The listing builds one solid part. Answer for the finished solid, in the listing's coordinates (mm). Coordinates: 2 decimals unless noted, no trailing zeros. Loops run counter-clockwise (first coordinate to the right, second up) from the corner with the lowest first, then second, coordinate; pieces in that order, holes last. Notation, with made-up numbers: (-13.5, 55) - (19.5, 55) arc R19 ccw to (19.5, 90) - close; hole circle Ø8 at (5, -11). An arc over 180 degrees is marked (long way). Put each result on its own line as item: value.
```python
from build123d import *

# Parameters (mm, degrees)
F1_DEPTH = 6


with BuildPart() as f1:
    # F0 (on Right) → F1 (new body)
    with BuildSketch(Plane.YZ):
        Polygon((9.433792, 157.218419), (-47.5, 157.218419), (-47.5, 130.369142), (-32.5, 130.369142), (-32.5, 142.218419), (9.433792, 142.218419), align=None)
        Polygon((62.5, 157.218419), (9.433792, 157.218419), (9.433792, 142.218419), (47.5, 142.218419), (47.5, 129.836887), (62.5, 129.836887), align=None)
        Polygon((-32.5, 130.369142), (-47.5, 130.369142), (-47.5, -62.781581), (62.5, -62.781581), (62.5, 129.836887), (47.5, 129.836887), (47.5, 119.718419), (-32.5, 119.718419), align=None)
        Polygon((-22.5, -19.281581), (-22.5, -22.781581), (-22.5, -26.281581), (-32.5, -26.281581), (-32.5, -19.281581), align=None, mode=Mode.SUBTRACT)
        Polygon((12.5, -19.281581), (12.5, -22.781581), (12.5, -26.281581), (2.5, -26.281581), (2.5, -22.781581), (2.5, -19.281581), align=None, mode=Mode.SUBTRACT)
        Polygon((37.5, -22.781581), (37.5, -19.281581), (47.5, -19.281581), (47.5, -26.281581), (37.5, -26.281581), align=None, mode=Mode.SUBTRACT)
        Polygon((-22.5, 55.718419), (-22.5, 52.218419), (-22.5, 48.718419), (-32.5, 48.718419), (-32.5, 55.718419), align=None, mode=Mode.SUBTRACT)
        Polygon((-22.5, 102.218419), (-22.5, 98.718419), (-32.5, 98.718419), (-32.5, 105.718419), (-22.5, 105.718419), align=None, mode=Mode.SUBTRACT)
        Polygon((12.5, 55.718419), (12.5, 52.218419), (12.5, 48.718419), (2.5, 48.718419), (2.5, 52.218419), (2.5, 55.718419), align=None, mode=Mode.SUBTRACT)
        Polygon((37.5, 52.218419), (37.5, 55.718419), (47.5, 55.718419), (47.5, 48.718419), (37.5, 48.718419), align=None, mode=Mode.SUBTRACT)
        Polygon((2.5, 98.718419), (2.5, 102.218419), (2.5, 105.718419), (12.5, 105.718419), (12.5, 102.218419), (12.5, 98.718419), align=None, mode=Mode.SUBTRACT)
        Polygon((37.5, 98.718419), (37.5, 102.218419), (37.5, 105.718419), (47.5, 105.718419), (47.5, 98.718419), align=None, mode=Mode.SUBTRACT)
    extrude(amount=F1_DEPTH)


solid = f1.part
```
1) The part is cut by section C-C (x = 3.3). State how many separate pieces and enclosed holes the cut face has, and give its area (3 significant figures).
Found:
separate pieces: 1
enclosed holes: 10
area: 21,800 mm^2
2) The part is cut by section A-A (y = 6). Give the vertices of the cut face in (x, z).
Found:
outline: (0, -62.78) - (6, -62.78) - (6, -26.28) - (0, -26.28) - close; (0, -19.28) - (6, -19.28) - (6, 48.72) - (0, 48.72) - close; (0, 55.72) - (6, 55.72) - (6, 98.72) - (0, 98.72) - close; (0, 105.72) - (6, 105.72) - (6, 119.72) - (0, 119.72) - close; (0, 142.22) - (6, 142.22) - (6, 157.22) - (0, 157.22) - close
3) Straight lines are drawn through the part: L1, parallel to Z at x = 3.15, y = 12; L2, parallel to Z at x = 3.9, y = 21.5. For each, find the intervals that lie inside material, in ascending order. Write a range as [from, to].
Found:
L1: z = [-62.78, -26.28], [-19.28, 48.72], [55.72, 98.72], [105.72, 119.72], [142.22, 157.22]
L2: z = [-62.78, 119.72], [142.22, 157.22]
4) The part is cut by section B-B (y = 21). Give the vertices of the cut face in (x, z).
Found:
outline: (0, -62.78) - (6, -62.78) - (6, 119.72) - (0, 119.72) - close; (0, 142.22) - (6, 142.22) - (6, 157.22) - (0, 157.22) - close
5) For a pull along Y with two mould halves and no side action, classify faces 1 (the face through (3, 2.5, -23)), 2 (the face through (3, -47.5, 49)) as pulls with the +Y half, pulls with the -Y half, needs draft (parallel to the pull), parting line crosses it, or undercut.
Found:
face 1: undercut
face 2: pulls with the -Y half
6) This flat-tipped pin is pushed along its axis until it touches: pin 1 (5 mm diameter, centred on y = 23.5, z = 122, fed in from -X). Where does it stop, or does it pass through?
Found:
pin 1: stops at x = 0
